Verification items for the finished model (mm, model axes). A direction names the side the tool comes from. Coordinates: 2 decimals unless noted, no trailing zeros. Order: outer loops, then holes, each group sorted by start corner. A loop starts at its lowest first (then second) coordinate and runs counter-clockwise, first axis right, second up. Notation, with made-up numbers: M 85,-9.5 L 94,-9.5 A25 ccw 94,6.5 Z; hole C 69.5,-18.75 d5. An arc over 180 degrees is marked long. Return JSON: item names as keys, results as strings. Group by question number.
Q1. Section check B-B, the plane x = 14.5. Enter the section's corners in (y, z), then the cut area to 3 significant figures.
Q2. Go/stop test with flat-tipped pins: pin 1 Ø12 at (x, y) = (14, 16.5) entering from +Z; pin 2 Ø6 at (x, z) = (36.42, -141.02) entering from +Y; pin 3 Ø10.5 at (x, y) = (5, 22.5) entering from -Z. Record where each tip stops, or that it passes through.
Q3. Thickness scan on probe 1 along X at (y, z) = (38.5, -96.5); probe 2 along Z at (x, y) = (-3, 23.5); probe 3 along Y at (x, z) = (35, 15). Record the ranges inside material, lowest first.
Q4. Section check C-C, the plane z = -59.5. Enter the section's corners in (x, y).
Q5. Access from +Z, -Z, +X, -X, +Y, -Y to the whole of each face (thin tool, end or side, straight path). Record for faces 1 (the face through (5, 24, -130.017)), 2 (the face through (-21.73, 2.96, 32.68)).
Q6. Mould release check, pull along Z, two halves, no side actions. Record for faces 3 (the face through (7, 0, -52)), 4 (the face through (6, 5.994, -55)), 5 (the face through (-33.323, 23.5, 26.355)), 6 (the face through (6, 3, -148.026)): pulls with the +Z half, pulls with the -Z half, needs draft (parallel to the pull), parting line crosses it, or undercut.
Autodesk Inventor part; units mm, degrees
ref_plane "YZ Plane" through (0, 0, 0) normal (1, 0, 0) x (0, 1, 0)
ref_plane "XZ Plane" through (0, 0, 0) normal (0, 1, 0) x (-1, 0, 0)
ref_plane "XY Plane" through (0, 0, 0) normal (0, 0, 1) x (1, 0, 0)
sketch "Sketch1" plane through (0, 0, 0) normal (0, 1, 0) x (-1, 0, 0)
  line L0 (-41.2899, 41.3823) -> (28.4387, 41.3823)
  line L1 (34.2779, 28.6823) -> (34.2779, -135.3255)
  line L2 (28.4387, -148.0255) -> (-41.2899, -148.0255)
  line L3 (-47.1291, -135.3255) -> (-47.1291, 28.6823)
  line L4 (-47.1291, 28.6823) -> (34.2779, 28.6823)
  line L5 (-47.1291, -135.3255) -> (34.2779, -135.3255)
  line L6 (34.2779, -135.3255) -> (31.5055, -145.6722)
  line L7 (-47.1291, -135.3255) -> (-44.3567, -145.6722)
  line L8 (-47.1291, 28.6823) -> (-44.3567, 39.0291)
  line L9 (34.2779, 28.6823) -> (31.5055, 39.0291)
  arc A0 (-44.3567, -145.6722) -> (-41.2899, -148.0255) centre (-41.2899, -144.8505) ccw
  arc A1 (28.4387, -148.0255) -> (31.5055, -145.6722) centre (28.4387, -144.8505) ccw
  arc A2 (31.5055, 39.0291) -> (28.4387, 41.3823) centre (28.4387, 38.2073) ccw
  arc A3 (-41.2899, 41.3823) -> (-44.3567, 39.0291) centre (-41.2899, 38.2073) ccw
  circle A4 centre (-36.423, -141.0151) radius 2.5019
  circle A5 centre (23.5718, -141.0151) radius 2.5019
  circle A6 centre (-36.423, 34.3719) radius 2.5019
  circle A7 centre (23.5718, 34.3719) radius 2.5019
  line L10 (-6.4256, 41.3823) -> (-6.4256, -148.0255) construction
  point P0 (0, 0)
  dimension "d2" = 12.7
  dimension "d3" = 12.7
  dimension "d4" = 15
  dimension "d5" = 15
  dimension "d6" = 15
  dimension "d7" = 81.407
  dimension "d8" = 189.4078
  dimension "d9" = 3.175
  dimension "d10" = 7.0104
  dimension "d11" = 7.0104
  dimension "d12" = 7.0104
  dimension "d13" = 7.0104
  dimension "d14" = 59.9948
  dimension "d15" = 59.9948
  dimension "d16" = 5.0038
  dimension "d17" = 5.0038
  dimension "d18" = 5.0038
  dimension "d19" = 5.0038
  dimension "d20" = 29.9974
  dimension "d21" = 29.9974
extrude "Extrusion1" add sketch "Sketch1" along normal blind 5.9944
sketch "Sketch2" plane through (0, 5.9944, 0) normal (0, 1, 0) x (1, 0, 0)
  line L0 (47.1291, -28.6823) -> (47.1291, 135.3255)
  line L1 (41.2899, 148.0255) -> (-28.4387, 148.0255)
  line L2 (-34.2779, 135.3255) -> (-34.2779, -28.6823)
  line L3 (-31.1029, 133.9285) -> (43.9541, 133.9285)
  line L4 (47.1291, 130.7535) -> (47.1291, -24.0849)
  line L5 (43.9541, -27.2599) -> (-31.1029, -27.2599)
  line L6 (-34.2779, -24.0849) -> (-34.2779, 130.7535)
  arc A0 (-34.2779, -24.0849) -> (-31.1029, -27.2599) centre (-31.1029, -24.0849) ccw
  arc A1 (43.9541, -27.2599) -> (47.1291, -24.0849) centre (43.9541, -24.0849) ccw
  arc A2 (47.1291, 130.7535) -> (43.9541, 133.9285) centre (43.9541, 130.7535) ccw
  arc A3 (-31.1029, 133.9285) -> (-34.2779, 130.7535) centre (-31.1029, 130.7535) ccw
  point P0 (0, 0)
  point P1 (-34.2779, 133.9285)
  point P2 (47.1291, -27.2599)
  dimension "d25" = 161.1884
  dimension "d26" = 14.097
  dimension "d27" = 3.175
extrude "Extrusion2" add sketch "Sketch2" along normal blind 35.5092
sketch "Sketch3" plane through (0, 41.5036, 0) normal (0, 1, 0) x (1, 0, 0)
  line L0 (-34.2779, 130.7535) -> (-34.2779, -24.0849)
  line L1 (43.9541, 133.9285) -> (-31.1029, 133.9285)
  line L2 (42.9, 118.3456) -> (42.9, -11.2706)
  line L3 (-30.0488, -11.2706) -> (-30.0488, 118.3456)
  line L4 (-19.4443, 130.0169) -> (30.4413, 130.0169)
  line L5 (30.4413, -22.9419) -> (-19.4443, -22.9419)
  arc A0 (33.6163, 126.8419) -> (30.4413, 130.0169) centre (30.4413, 126.8419) ccw
  arc A1 (-19.4443, 130.0169) -> (-22.6193, 126.8419) centre (-19.4443, 126.8419) ccw
  arc A2 (-22.6193, -19.7669) -> (-19.4443, -22.9419) centre (-19.4443, -19.7669) ccw
  arc A3 (30.4413, -22.9419) -> (33.6163, -19.7669) centre (30.4413, -19.7669) ccw
  arc A4 (-30.0488, -11.2706) -> (-26.8738, -14.4456) centre (-26.8738, -11.2706) ccw
  arc A5 (-26.8738, 121.5206) -> (-30.0488, 118.3456) centre (-26.8738, 118.3456) ccw
  arc A6 (42.9, 118.3456) -> (39.725, 121.5206) centre (39.725, 118.3456) ccw
  arc A7 (39.725, -14.4456) -> (42.9, -11.2706) centre (39.725, -11.2706) ccw
  line L6 (33.6163, 126.8419) -> (33.6163, 126.0164)
  line L7 (33.6163, -18.9414) -> (33.6163, -19.7669)
  line L8 (-22.6193, -19.7669) -> (-22.6193, -18.9414)
  line L9 (-22.6193, 126.0164) -> (-22.6193, 126.8419)
  line L10 (39.725, -14.4456) -> (38.1121, -14.4456)
  line L11 (-27.1151, -14.4456) -> (-26.8738, -14.4456)
  line L12 (-26.8738, 121.5206) -> (-27.1151, 121.5206)
  line L13 (38.1121, 121.5206) -> (39.725, 121.5206)
  arc A8 (38.1121, -14.4456) -> (33.6163, -18.9414) centre (38.1121, -18.9414) ccw
  arc A9 (33.6163, 126.0164) -> (38.1121, 121.5206) centre (38.1121, 126.0164) ccw
  arc A10 (-27.1151, 121.5206) -> (-22.6193, 126.0164) centre (-27.1151, 126.0164) ccw
  arc A11 (-22.6193, -18.9414) -> (-27.1151, -14.4456) centre (-27.1151, -18.9414) ccw
  point P0 (0, 0)
  point P1 (42.9, 76.4991)
  point P2 (42.9, 110.1795)
  point P3 (-30.0488, 76.4991)
  point P4 (-22.7463, 130.0169)
  point P5 (33.6163, -22.9419)
  point P6 (33.6163, 130.0169)
  dimension "d30" = 56.3626
  dimension "d32" = 152.9588
  dimension "d35" = 72.9488
  dimension "d36" = 4.2291
  dimension "d37" = 3.9116
  dimension "d38" = 3.175
  dimension "d39" = 4.4958
  dimension "d42" = 135.9662
  dimension "d43" = 8.4963
extrude "Extrusion3" cut sketch "Sketch3" against normal blind 35.5092
properties part number "NEAMBoxLarge"
Numbers:
{
 "1": {"outline": "M 0,-148.03 L 5.99,-148.03 L 5.99,-133.93 L 41.5,-133.93 L 41.5,-130.02 L 5.99,-130.02 L 5.99,22.94 L 41.5,22.94 L 41.5,27.26 L 5.99,27.26 L 5.99,41.38 L 0,41.38 Z", "area": "1,430 mm2"},
 "2": {"pin 1": "stops at z = 27.26", "pin 2": "stops at y = 5.99", "pin 3": "stops at z = -133.93"},
 "3": {"probe 1": "x = -34.28 to -30.05, 42.9 to 47.13", "probe 2": "z = -133.93 to -130.02, 22.94 to 27.26", "probe 3": "y = 0 to 5.99"},
 "4": {"outline": "M -34.28,0 L 47.13,0 L 47.13,41.5 L 42.9,41.5 L 42.9,5.99 L -30.05,5.99 L -30.05,41.5 L -34.28,41.5 Z"},
 "5": {"face 1": "+Y", "face 2": "+Y, -Y"},
 "6": {"face 3": "needs draft", "face 4": "undercut", "face 5": "pulls with the +Z half", "face 6": "pulls with the -Z half"}
}
